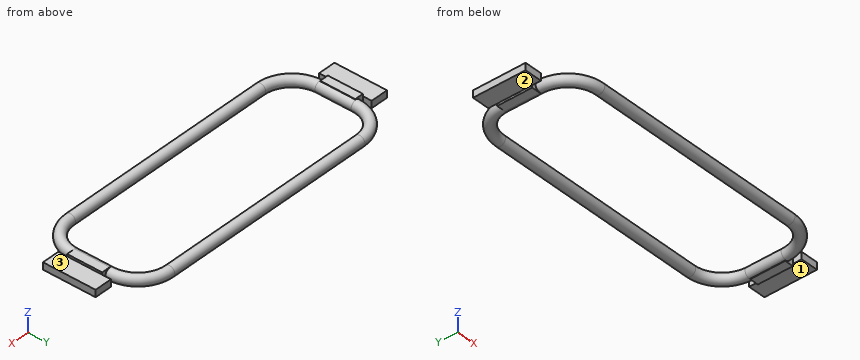
```python
from build123d import *

# Parameters (mm, degrees)
SKETCH1_W           = 100
SKETCH1_H           = 75
SKETCH1_H_2         = 150
BOSS_EXTRUDE1_DEPTH = 20
SKETCH4_W           = 50
SKETCH4_H           = 150
BOSS_EXTRUDE3_DEPTH = 6.25
SKETCH5_W           = 50
SKETCH5_H           = 150
BOSS_EXTRUDE4_DEPTH = 6.25
SKETCH21_W          = 850
SKETCH21_H          = 32.5
CUT_EXTRUDE2_DEPTH  = 25
CUT_EXTRUDE3_START  = -150
SKETCH21_2_W        = 850
SKETCH21_2_H        = 32.5
CUT_EXTRUDE3_DEPTH  = 25
SWEEP1_PROFILE_R    = 15
CUT_EXTRUDE1_DEPTH  = 50


with BuildPart() as part:
    # Sketch1 → Boss-Extrude1 (new body)
    with BuildSketch(Plane.XY):
        with Locations((-850, 37.5)):
            Rectangle(SKETCH1_W, SKETCH1_H)
        with Locations((-850, -37.5)):
            Rectangle(SKETCH1_W, SKETCH1_H)
        Rectangle(SKETCH1_W, SKETCH1_H_2)
    extrude(amount=BOSS_EXTRUDE1_DEPTH)

    # Sketch4 → Boss-Extrude3 (add)
    with BuildSketch(Plane(origin=(0, 0, 0), x_dir=(-1, 0, 0), z_dir=(0, 0, -1))):
        with Locations((25, 0)):
            Rectangle(SKETCH4_W, SKETCH4_H)
        with Locations((825, 0)):
            Rectangle(SKETCH4_W, SKETCH4_H)
    extrude(amount=BOSS_EXTRUDE3_DEPTH)

    # Sketch5 → Boss-Extrude4 (add)
    with BuildSketch(Plane.XY.offset(20)):
        with Locations((-825, 0)):
            Rectangle(SKETCH5_W, SKETCH5_H)
        with Locations((-25, 0)):
            Rectangle(SKETCH5_W, SKETCH5_H)
    extrude(amount=BOSS_EXTRUDE4_DEPTH)

    # Sketch21 → Cut-Extrude2 (cut)
    with BuildSketch(Plane(origin=(0, 75, 0), x_dir=(1, 0, 0), z_dir=(0, 1, 0))):
        with Locations((-425, -10)):
            Rectangle(SKETCH21_W, SKETCH21_H)
    extrude(amount=-CUT_EXTRUDE2_DEPTH, mode=Mode.SUBTRACT)

    # Sketch21<2> → Cut-Extrude3 (cut)
    with BuildSketch(Plane(origin=(0, 75, 0), x_dir=(1, 0, 0), z_dir=(0, 1, 0)).offset(CUT_EXTRUDE3_START)):
        with Locations((-425, -10)):
            Rectangle(SKETCH21_2_W, SKETCH21_2_H)
    extrude(amount=CUT_EXTRUDE3_DEPTH, mode=Mode.SUBTRACT)

    # Sweep1: sweep along a path in Sketch6
    with BuildLine(Plane.XY.offset(10)) as sweep1_path:
        Line((-115, -141.504877042), (-735, -141.504877042))
        ThreePointArc((-735, -141.504877042), (-798.639610307, -115.144487349), (-825, -51.504877042))
        Line((-825, -51.504877042), (-825, 51.504877042))
        ThreePointArc((-825, 51.504877042), (-798.639610307, 115.144487349), (-735, 141.504877042))
        Line((-735, 141.504877042), (-115, 141.504877042))
        ThreePointArc((-115, 141.504877042), (-51.360389693, 115.144487349), (-25, 51.504877042))
        Line((-25, 51.504877042), (-25, -51.504877042))
        ThreePointArc((-25, -51.504877042), (-51.360389693, -115.144487349), (-115, -141.504877042))
    # Sweep1 profile (on start of the path) → Sweep1 (sweep)
    with BuildSketch(Plane(origin=(-115, -141.504877042, 10), x_dir=(0, 0, -1), z_dir=(-1, 0, 0))):
        Circle(SWEEP1_PROFILE_R)
    sweep(path=sweep1_path.line)

    # Sketch19 → Cut-Extrude1 (cut, symmetric)
    with BuildSketch(Plane(origin=(0, 0, 0), x_dir=(1, 0, 0), z_dir=(0, 1, 0))):
        with BuildLine():
            Line((-825, -26.25), (-825, -25))
            ThreePointArc((-825, -25), (-810, -10), (-825, 5))
            Line((-825, 5), (-825, 6.25))
            Line((-825, 6.25), (-800, 6.25))
            Line((-800, 6.25), (-800, -26.25))
            Line((-800, -26.25), (-825, -26.25))
        make_face()
        with BuildLine():
            Line((-50, -26.25), (-25, -26.25))
            Line((-25, -26.25), (-25, -25))
            ThreePointArc((-25, -25), (-40, -10), (-25, 5))
            Line((-25, 5), (-25, 6.25))
            Line((-25, 6.25), (-50, 6.25))
            Line((-50, 6.25), (-50, -26.25))
        make_face()
    extrude(amount=CUT_EXTRUDE1_DEPTH, both=True, mode=Mode.SUBTRACT)


solid = part.part
```
Model file for the job. Use its own axes, mm. Face numbers are marked on the shaded views. A direction names the side the tool comes from. Coordinates: 2 decimals unless noted, no trailing zeros. Order: outer loops, then holes, each group sorted by start corner. A loop starts at its lowest first (then second) coordinate and runs counter-clockwise, first axis right, second up. Notation, with made-up numbers: (-25, -39.75) - (15, -39.75) arc R15 cw to (15, -32.75) - close; hole circle Ø11 at (0, -34.5). An arc over 180 degrees is marked (long way). Return JSON: item names as keys, results as strings. Group by question number.
1) Tool access for the marked faces 1, 2 and 3: list every direction of +Z, -Z, +X, -X, +Y, -Y with a clear straight run to the whole face (end or side of a thin tool).
2) Probe line 1 (X direction, y = -55, z = 9); line 2 (Y direction, x = -718, z = 8); line 3 (Y direction, x = -420, z = 9). List the from-to ranges inside material, lowest first. Write a range as from..to.
3) Flat gauge pins, fed straight in: P1, Ø12.5, axis at x = -18.5, z = 10.5, coming from the -Y side; P2, Ø0.6, axis at y = -24.5, z = 25.5, coming from the +X side; P3, Ø0.6, axis at y = 16, z = 25.5, coming from the -X side. Where does each tip first touch, or does it go through?
4) Saw through at C-C, the plane x = -566. Write the cut outline in (y, z).
5) Saw through at A-A, the plane y = -19.5. Write the cut outline in (x, z), plus the area to 3 significant figures.
6) Saw through at D-D, the plane y = 61.5. Count the separate pieces of the cut face and the enclosed holes in it, plus the area to 3 significant figures.
Values found:
{
 "1": {"face 1": "-Z, +X, +Y, -Y", "face 2": "-Z, -X, +Y, -Y", "face 3": "+Z, +X, +Y, -Y"},
 "2": {"line 1": "x = -900..-850, -839.91..-809.95, -40.05..-10.09, 0..50", "line 2": "y = -156.37..-126.64, 126.64..156.37", "line 3": "y = -156.47..-126.54, 126.54..156.47"},
 "3": {"P1": "stops at y = -105.16", "P2": "stops at x = 0", "P3": "stops at x = -850"},
 "4": {"outline": "circle Ø30 at (-141.5, 10); circle Ø30 at (141.5, 10)"},
 "5": {"outline": "(-900, 0) - (-850, 0) - (-850, -6.25) - (-825, -6.25) - (-825, -5) arc R15 ccw to (-825, 25) - (-825, 26.25) - (-850, 26.25) - (-850, 20) - (-900, 20) - close; (-25, -6.25) - (0, -6.25) - (0, 0) - (50, 0) - (50, 20) - (0, 20) - (0, 26.25) - (-25, 26.25) - (-25, 25) arc R15 ccw to (-25, -5) - close", "area": "4,330 mm²"},
 "6": {"separate pieces": "4", "enclosed holes": "0", "area": "3,420 mm²"}
}
